Read the model definition and answer for the solid it produces. Units are mm, in the model's axes. A direction names the side the tool comes from. Coordinates: 2 decimals unless noted, no trailing zeros. Write each loop counter-clockwise with the first axis right and the second up, starting at its lowest first coordinate (ties: lowest second). Pieces come first, ordered by that corner, then holes.
(1) Given pin 1 (3 mm diameter, centred on x = 12.5, y = 5.5, fed in from +Z); pin 2 (5.5 mm diameter, centred on y = 2.5, z = -2.5, fed in from +X); pin 3 (1 mm diameter, centred on x = 12.5, z = -1, fed in from +Y), each flat-ended and moving along its own axis, determine where each tip first touches the part or whether it passes through.
(2) Section A-A on x = 24 is taken. Write down the section's boundary in (y, z).
(3) Find the intervals of material crossed by probe 1 along Z at (x, y) = (30, 4.5); probe 2 along Z at (x, y) = (6, 4.5); probe 3 along X at (y, z) = (7.25, -4), in increasing order.
(4) Which of the six approach directions +Z, -Z, +X, -X, +Y, -Y give full straight-line access (tool end or side, diameter ignored) to faces 1 (the cylindrical face through (29.9, 0.7, -2.5)), 2 (the flat face through (36.9, 5, 0))?
from build123d import *

# Parameters (mm, degrees)
FILETE1_R = 0.2


with BuildPart() as part:
    # Esboço1 → Revolução1 (revolve)
    with BuildSketch(Plane.XY, mode=Mode.PRIVATE) as revolu_o1_sk:
        with BuildLine():
            Line((0, 4.678862418), (0, 10.228862418))
            Line((0, 10.228862418), (1.4, 10.228862418))
            Line((1.4, 10.228862418), (1.4, 9.478862418))
            Line((1.4, 9.478862418), (28.92, 9.478862418))
            ThreePointArc((28.92, 9.478862418), (28.976568542, 9.455430961), (29, 9.398862418))
            Line((29, 9.398862418), (29, 9.378862418))
            Line((29, 9.378862418), (31, 9.378862418))
            Line((31, 9.378862418), (31, 9.300321604))
            ThreePointArc((31, 9.300321604), (31.088208078, 9.049750661), (31.313928988, 8.909691624))
            Line((31.313928988, 8.909691624), (36.9, 7.678862418))
            Line((36.9, 7.678862418), (36.9, 4.678862418))
            Line((36.9, 4.678862418), (0, 4.678862418))
        make_face()
    revolve(revolu_o1_sk.sketch.rotate(Axis((36.9, 4.678862418, 0), (-1, 0, 0)), 90), axis=Axis((36.9, 4.678862418, 0), (-1, 0, 0)))

    # Filete1
    filete1_edges = [part.edges().sort_by_distance(p)[0] for p in [
        (31, 4.678862418, 4.7),
    ]]
    fillet(filete1_edges, radius=FILETE1_R)


solid = part.part
Response:
1. pin 1: stops at z = 4.8
1. pin 2: stops at x = 36.9
1. pin 3: stops at y = 9.45
2. outline: circle Ø9.6 at (4.68, 0)
3. probe 1: z = -4.7 to 4.7
3. probe 2: z = -4.8 to 4.8
3. probe 3: x = 0 to 28.99
4. face 1: +X
4. face 2: +Z, -Z, +X, +Y, -Y
